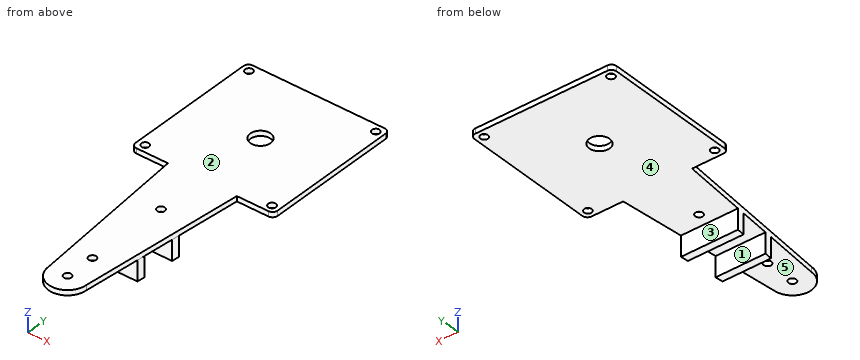
```python
from build123d import *

# Parameters (mm, degrees)
SKETCH2_R           = 1.5
BOSS_EXTRUDE1_DEPTH = 2
SKETCH3_R           = 4
CUT_EXTRUDE1_DEPTH  = 10
BOSS_EXTRUDE2_DEPTH = 8
SKETCH5_R           = 1.5
CUT_EXTRUDE2_DEPTH  = 2
SKETCH6_R           = 7.5
BOSS_EXTRUDE3_DEPTH = 2
SKETCH7_R           = 1.5
CUT_EXTRUDE3_DEPTH  = 2


with BuildPart() as part:
    # Sketch2 → Boss-Extrude1 (new body)
    with BuildSketch(Plane.XY):
        with BuildLine():
            Line((-13.59375, -28), (-26, -28))
            ThreePointArc((-26, -28), (-27.414213562, -27.414213562), (-28, -26))
            Line((-28, -26), (-28, 26))
            ThreePointArc((-28, 26), (-27.414213562, 27.414213562), (-26, 28))
            Line((-26, 28), (26, 28))
            ThreePointArc((26, 28), (27.414213562, 27.414213562), (28, 26))
            Line((28, 26), (28, -26))
            ThreePointArc((28, -26), (27.414213562, -27.414213562), (26, -28))
            Line((26, -28), (13.555660481, -28))
            Line((13.555660481, -28), (7.5, -93))
            Line((7.5, -93), (-7.5, -93))
            Line((-7.5, -93), (-13.59375, -28))
        make_face()
        with Locations((25, 25)):
            Circle(SKETCH2_R, mode=Mode.SUBTRACT)
        with Locations((25, -25)):
            Circle(SKETCH2_R, mode=Mode.SUBTRACT)
        with Locations((-25, -25)):
            Circle(SKETCH2_R, mode=Mode.SUBTRACT)
        with Locations((-25, 25)):
            Circle(SKETCH2_R, mode=Mode.SUBTRACT)
    extrude(amount=BOSS_EXTRUDE1_DEPTH)

    # Sketch3 → Cut-Extrude1 (cut)
    with BuildSketch(Plane.XY.offset(2)):
        Circle(SKETCH3_R)
    extrude(amount=-CUT_EXTRUDE1_DEPTH, mode=Mode.SUBTRACT)

    # Sketch4 → Boss-Extrude2 (add)
    with BuildSketch(Plane(origin=(0, 0, 0), x_dir=(-1, 0, 0), z_dir=(0, 0, -1))):
        Polygon((-11.226560296, -53), (-10.96875, -56), (10.96875, -56), (11.25, -53), align=None)
        Polygon((-9.84375, -68), (-9.5625, -71), (9.5625, -71), (9.84375, -68), align=None)
    extrude(amount=BOSS_EXTRUDE2_DEPTH)

    # Sketch5 → Cut-Extrude2 (cut)
    with BuildSketch(Plane(origin=(0, 0, 0), x_dir=(-1, 0, 0), z_dir=(0, 0, -1))):
        with Locations((0, -48)):
            Circle(SKETCH5_R)
        with Locations((0, -81)):
            Circle(SKETCH5_R)
    extrude(amount=-CUT_EXTRUDE2_DEPTH, mode=Mode.SUBTRACT)

    # Sketch6 → Boss-Extrude3 (add)
    with BuildSketch(Plane(origin=(0, 0, 0), x_dir=(-1, 0, 0), z_dir=(0, 0, -1))):
        with Locations((0, -93)):
            Circle(SKETCH6_R)
    extrude(amount=-BOSS_EXTRUDE3_DEPTH)

    # Sketch7 → Cut-Extrude3 (cut)
    with BuildSketch(Plane.XY.offset(2)):
        with Locations((0, -93)):
            Circle(SKETCH7_R)
    extrude(amount=-CUT_EXTRUDE3_DEPTH, mode=Mode.SUBTRACT)


solid = part.part
```
The listing builds one solid part. Answer for the finished solid, in the listing's coordinates (mm). Face numbers are marked on the shaded views. A direction names the side the tool comes from. Give positions to 0.01 mm unless a question says otherwise; leave off trailing zeros. Loops run counter-clockwise (first coordinate to the right, second up) from the corner with the lowest first, then second, coordinate; pieces in that order, holes last. Notation, with made-up numbers: M 46.25,5.25 L 82.25,5.25 A32 cw 82.25,42.25 Z; hole C 2.25,43.25 d1. An arc over 180 degrees is marked long. One line per item, written item: value.
1. For a pull along Y with two mould halves and no side action, classify the marked faces 1, 2 and 3 as pulls with the +Y half, pulls with the -Y half, needs draft (parallel to the pull), parting line crosses it, or undercut.
Found:
face 1: undercut
face 2: needs draft
face 3: pulls with the +Y half
2. Each of these flat-tipped pins is pushed along its axis until it touches: P1, Ø4, axis at x = -4.5, z = -3, coming from the -Y side; P2, Ø4, axis at x = -25, y = -25, coming from the -Z side; P3, Ø2, axis at x = -19, z = 0.5, coming from the -Y side. Where does it stop, or does it pass through?
Found:
P1: y = -71
P2: z = 0
P3: y = -28
3. Section A-A on z = -1.75 is taken. Determine the outline of the cut face in (x, y).
Found:
outline: M -11.25,-53 L -10.97,-56 L 10.97,-56 L 11.23,-53 Z; M -9.84,-68 L -9.56,-71 L 9.56,-71 L 9.84,-68 Z
4. Section C-C on y = -89 is taken. Determine the outline of the cut face in (x, z) (3 decimals).
Found:
outline: M -7.875,0 L 7.873,0 L 7.873,2 L -7.875,2 Z
5. Find the intervals of material crossed by probe 1 along Y at (x, z) = (25, 1.45); probe 2 along Y at (x, z) = (0, 0.95); probe 3 along Y at (x, z) = (-4, -2.5), in increasing order.
Found:
probe 1: -28 to -26.5, -23.5 to 23.5, 26.5 to 28
probe 2: -100.5 to -94.5, -91.5 to -82.5, -79.5 to -49.5, -46.5 to -4, 4 to 28
probe 3: -71 to -68, -56 to -53
6. Section D-D on y = -42 is taken. Determine the outline of the cut face in (x, z).
Found:
outline: M -12.28,0 L 12.25,0 L 12.25,2 L -12.28,2 Z
7. For the marked faces 4 and 5, determine the directions among +Z, -Z, +X, -X, +Y, -Y from which every point of the face is accessible in a straight line to the end or side of a thin tool.
Found:
face 4: -Z, +X, -X, +Y
face 5: -Z, +X, -X, -Y
8. Section B-B on y = 0 is taken. Determine the outline of the cut face in (x, z).
Found:
outline: M -28,0 L -4,0 L -4,2 L -28,2 Z; M 4,0 L 28,0 L 28,2 L 4,2 Z
